CAD build for the part. Positions are in the model's coordinates, mm. A direction names the side the tool comes from. Round coordinates to 2 decimals unless told otherwise and drop trailing zeros. Order: outer loops, then holes, each group sorted by start corner. A loop starts at its lowest first (then second) coordinate and runs counter-clockwise, first axis right, second up. Notation, with made-up numbers: (17, 7) -> (24, 7) arc R21 cw to (24, 33) -> close; hole circle Ø5 at (38, 21.5). An arc over 180 degrees is marked (long way). Return JSON: item names as keys, results as strings. Group by question number.
Q1. Mould opens along X. For faces 1 (the conical face through (4.71, -8.38, -6.15)), 2 (the cylindrical face through (-2.806, -0.986, 1.641)), 3 (the flat face through (-2, 0, 2)) say: +X half, -X half, draft (parallel to the pull), parting line (faces both ways), or undercut.
Q2. Cut at C-C (y = -14.75). Write the cut outline in (x, z).
Q3. Probe line 1 along Z through (x, y) = (0, -15.85); line 2 along Z through (x, y) = (0, -14.5); line 3 along Y through (x, z) = (-5.5, -1). List the from-to ranges inside material, lowest first.
Q4. Flat gauge pins, fed straight in: pin 1 (1.6 mm diameter, centred on x = -3.5, z = 2.5, fed in from +Y); pin 2 (4 mm diameter, centred on x = -1.5, y = -12.5, fed in from +Z); pin 3 (1.5 mm diameter, centred on x = 4, y = -8.5, fed in from +Z). Where does each tip first touch, or does it go through?
Q5. Cut at A-A (x = 0). Write the cut outline in (y, z).
Q6. Cut at D-D (y = -1.75). Write the cut outline in (x, z).
Q7. Cut at B-B (z = 0). Write the cut outline in (x, y).
Q8. Which spindle directions (+Z, -Z, +X, -X, +Y, -Y) get a long thin tool onto all of the face, cutting with end or side? Do faces 4 (the cylindrical face through (2.192, -15.028, -4.214)), 5 (the cylindrical face through (-0.54, -8.38, -2.44)), 6 (the flat face through (3.01, -0.99, -3.18)). Say none if no direction does.
from build123d import *

# Parameters (mm, degrees)
F0_R     = 8
F0_R_2   = 2.5
F1_DEPTH = 17
F2_R     = 7
F2_R_2   = 4.75
F3_DEPTH = 4
F5_DEPTH = 2


with BuildPart() as f1:
    # F0 (on Front) → F1 (new body)
    with BuildSketch(Plane.XZ):
        Circle(F0_R)
        Circle(F0_R_2, mode=Mode.SUBTRACT)
    extrude(amount=F1_DEPTH)

    # F2 (on face) → F3 (cut)
    with BuildSketch(Plane.XZ.offset(17)):
        Circle(F2_R)
        Circle(F2_R_2, mode=Mode.SUBTRACT)
    extrude(amount=-F3_DEPTH, mode=Mode.SUBTRACT)

    # F4 (on face) → F5 (cut)
    with BuildSketch(Plane(origin=(0, 0, 0), x_dir=(-1, 0, 0), z_dir=(0, 1, 0))):
        with BuildLine():
            ThreePointArc((-3.223076, 0.417468), (-2.814583, 1.625), (-1.973076, 2.582532))
            Line((-1.973076, 2.582532), (-4.013494, 3.760567))
            ThreePointArc((-4.013494, 3.760567), (-4.76314, 2.75), (-5.263494, 1.595504))
            Line((-5.263494, 1.595504), (-3.223076, 0.417468))
        make_face()
        with BuildLine():
            Line((-3.223076, -0.417468), (-5.263494, -1.595504))
            ThreePointArc((-5.263494, -1.595504), (-4.76314, -2.75), (-4.013494, -3.760567))
            Line((-4.013494, -3.760567), (-1.973076, -2.582532))
            ThreePointArc((-1.973076, -2.582532), (-2.814583, -1.625), (-3.223076, -0.417468))
        make_face()
        with BuildLine():
            Line((1.973076, -2.582532), (4.013494, -3.760567))
            ThreePointArc((4.013494, -3.760567), (4.76314, -2.75), (5.263494, -1.595504))
            Line((5.263494, -1.595504), (3.223076, -0.417468))
            ThreePointArc((3.223076, -0.417468), (2.814583, -1.625), (1.973076, -2.582532))
        make_face()
        with BuildLine():
            Line((3.223076, 0.417468), (5.263494, 1.595504))
            ThreePointArc((5.263494, 1.595504), (4.76314, 2.75), (4.013494, 3.760567))
            Line((4.013494, 3.760567), (1.973076, 2.582532))
            ThreePointArc((1.973076, 2.582532), (2.814583, 1.625), (3.223076, 0.417468))
        make_face()
    extrude(amount=-F5_DEPTH, mode=Mode.SUBTRACT)

    # F6 (on Right) → F7 (revolve, cut)
    with BuildSketch(Plane.YZ):
        Polygon((0, 8), (-17, 8), (0, 7.5), align=None)
    revolve(axis=Axis((0, -3.680971, 0), (0, -1, 0)), mode=Mode.SUBTRACT)


solid = f1.part
Solution:
{
 "1": {"face 1": "parting line", "face 2": "undercut", "face 3": "draft"},
 "2": {"outline": "circle Ø15.87 at (0, 0); circle Ø9.5 at (0, 0); hole circle Ø14 at (0, 0); hole circle Ø5 at (0, 0)"},
 "3": {"line 1": "z = -7.97 to -7, -4.75 to -2.5, 2.5 to 4.75, 7 to 7.97", "line 2": "z = -7.93 to -7, -4.75 to -2.5, 2.5 to 4.75, 7 to 7.93", "line 3": "y = -13 to 0"},
 "4": {"pin 1": "stops at y = -2", "pin 2": "stops at z = 7.91", "pin 3": "stops at z = 7.04"},
 "5": {"outline": "(-17, -8) -> (0, -7.5) -> (0, -2.5) -> (-17, -2.5) -> (-17, -4.75) -> (-13, -4.75) -> (-13, -7) -> (-17, -7) -> close; (-17, 2.5) -> (0, 2.5) -> (0, 7.5) -> (-17, 8) -> (-17, 7) -> (-13, 7) -> (-13, 4.75) -> (-17, 4.75) -> close"},
 "6": {"outline": "circle Ø15.1 at (0, 0); hole (-5.26, -1.6) arc R5.5 ccw to (-4.01, -3.76) -> (-1.97, -2.58) arc R3.25 cw to (-3.22, -0.42) -> close; hole (-5.26, 1.6) -> (-3.22, 0.42) arc R3.25 cw to (-1.97, 2.58) -> (-4.01, 3.76) arc R5.5 ccw to start; hole circle Ø5 at (0, 0); hole (1.97, -2.58) -> (4.01, -3.76) arc R5.5 ccw to (5.26, -1.6) -> (3.22, -0.42) arc R3.25 cw to start; hole (1.97, 2.58) arc R3.25 cw to (3.22, 0.42) -> (5.26, 1.6) arc R5.5 ccw to (4.01, 3.76) -> close"},
 "7": {"outline": "(-8, -17) -> (-7, -17) -> (-7, -13) -> (-4.75, -13) -> (-4.75, -17) -> (-2.5, -17) -> (-2.5, 0) -> (-7.5, 0) -> close; (2.5, -17) -> (4.75, -17) -> (4.75, -13) -> (7, -13) -> (7, -17) -> (8, -17) -> (7.5, 0) -> (2.5, 0) -> close"},
 "8": {"face 4": "-Y", "face 5": "+Y, -Y", "face 6": "+Y"}
}
